```python
from build123d import *

# Parameters (mm, degrees)
BOSS_EXTRUDE1_DEPTH = 1.3
SKETCH2_W           = 6.25
SKETCH2_H           = 1
CUT_EXTRUDE1_DEPTH  = 128.618193671
SKETCH3_W           = 12
SKETCH3_H           = 1
SKETCH3_W_2         = 30
SKETCH3_W_3         = 14
SKETCH3_W_4         = 1
SKETCH3_H_2         = 8
CUT_EXTRUDE2_DEPTH  = 128.618193671
SKETCH4_W           = 1
SKETCH4_H           = 10
CUT_EXTRUDE3_DEPTH  = 128.618193671
SKETCH5_W           = 25
SKETCH5_H           = 1
SKETCH5_W_2         = 1
SKETCH5_H_2         = 20
CUT_EXTRUDE4_DEPTH  = 128.618193671
SKETCH6_W           = 1
SKETCH6_H           = 10
CUT_EXTRUDE5_DEPTH  = 128.618193671
SKETCH7_W           = 24
SKETCH7_H           = 0.5
SKETCH7_W_2         = 86
SKETCH7_W_3         = 18
BOSS_EXTRUDE2_DEPTH = 1.3
CUT_EXTRUDE6_DEPTH  = 128.618193671
SKETCH10_W          = 1
SKETCH10_H          = 40.53071679
BOSS_EXTRUDE3_DEPTH = 1.3


with BuildPart() as part:
    # Sketch1 → Boss-Extrude1 (new body)
    with BuildSketch(Plane(origin=(0, 0, 0), x_dir=(0, 0, -1), z_dir=(1, 0, 0))):
        with BuildLine():
            Line((81.367510562, 0), (81.367510562, 40))
            Line((81.367510562, 40), (68.86751224, 40))
            Line((68.86751224, 40), (68.86751224, 31.6))
            ThreePointArc((68.86751224, 31.6), (60.650673838, 32.5501447), (52.86751224, 35.350431081))
            ThreePointArc((52.86751224, 35.350431081), (27.570153703, 44.311585339), (0.86751224, 47))
            ThreePointArc((0.86751224, 47), (-29.363130095, 42.186071485), (-57.13248776, 29.304750955))
            ThreePointArc((-57.13248776, 29.304750955), (-60.244560512, 27.872141345), (-63.63248776, 27.362910487))
            ThreePointArc((-63.63248776, 27.362910487), (-91.690071427, 24.380332585), (-118.63248776, 16))
            ThreePointArc((-118.63248776, 16), (-117.739294054, 7.999999906), (-118.632489438, 0))
            Line((-118.632489438, 0), (-94.632489438, 0))
            ThreePointArc((-94.632489438, 0), (-76.632489438, 18), (-58.632489438, 0))
            Line((-58.632489438, 0), (27.367510562, 0))
            ThreePointArc((27.367510562, 0), (45.367510562, 18), (63.367510562, 0))
            Line((63.367510562, 0), (81.367510562, 0))
        make_face()
        with BuildLine():
            Line((-42.73248776, 29.304750955), (-2.13248776, 29.304750955))
            Line((-2.13248776, 29.304750955), (-2.13248776, 40.804750955))
            ThreePointArc((-2.13248776, 40.804750955), (-23.231125157, 37.874288199), (-42.73248776, 29.304750955))
        make_face(mode=Mode.SUBTRACT)
    extrude(amount=BOSS_EXTRUDE1_DEPTH)

    # Sketch2 → Cut-Extrude1 (cut, through all)
    with BuildSketch(Plane(origin=(1.3, 0, 0), x_dir=(0, 0, -1), z_dir=(1, 0, 0))):
        with Locations((75.242510562, 38)):
            Rectangle(SKETCH2_W, SKETCH2_H)
    extrude(amount=-CUT_EXTRUDE1_DEPTH, mode=Mode.SUBTRACT)

    # Sketch3 → Cut-Extrude2 (cut, through all)
    with BuildSketch(Plane(origin=(1.3, 0, 0), x_dir=(0, 0, -1), z_dir=(1, 0, 0))):
        with Locations((73.117510562, 1.75)):
            Rectangle(SKETCH3_W, SKETCH3_H)
        with Locations((6.367510562, 1.75)):
            Rectangle(SKETCH3_W_2, SKETCH3_H)
        with Locations((-105.632489438, 1.75)):
            Rectangle(SKETCH3_W_3, SKETCH3_H)
        Polygon((-90.165047606, 22.486285602), (-72.411906778, 25.457142507), (-72.246859172, 24.470856905), (-90, 21.5), align=None)
        with Locations((-107.132489438, 10.75)):
            Rectangle(SKETCH3_W_4, SKETCH3_H_2)
        Polygon((39.458953443, 39.317791271), (59.607847956, 30.484782164), (59.206347542, 29.568923322), (39.057453029, 38.40193243), align=None)
        with Locations((-33.632489438, 1.75)):
            Rectangle(SKETCH3_W_2, SKETCH3_H)
    extrude(amount=-CUT_EXTRUDE2_DEPTH, mode=Mode.SUBTRACT)

    # Sketch4 → Cut-Extrude3 (cut, through all)
    with BuildSketch(Plane(origin=(1.3, 0, 0), x_dir=(0, 0, -1), z_dir=(1, 0, 0))):
        with Locations((79.367510562, 15.75)):
            Rectangle(SKETCH4_W, SKETCH4_H)
    extrude(amount=-CUT_EXTRUDE3_DEPTH, mode=Mode.SUBTRACT)

    # Sketch5 → Cut-Extrude4 (cut, through all)
    with BuildSketch(Plane(origin=(1.3, 0, 0), x_dir=(0, 0, -1), z_dir=(1, 0, 0))):
        with Locations((3.867510562, 43.75)):
            Rectangle(SKETCH5_W, SKETCH5_H)
        with Locations((5.867510562, 22)):
            Rectangle(SKETCH5_W_2, SKETCH5_H_2)
    extrude(amount=-CUT_EXTRUDE4_DEPTH, mode=Mode.SUBTRACT)

    # Sketch6 → Cut-Extrude5 (cut, through all)
    with BuildSketch(Plane(origin=(1.3, 0, 0), x_dir=(0, 0, -1), z_dir=(1, 0, 0))):
        with Locations((-47.132489438, 12.25)):
            Rectangle(SKETCH6_W, SKETCH6_H)
    extrude(amount=-CUT_EXTRUDE5_DEPTH, mode=Mode.SUBTRACT)

    # Sketch7 → Boss-Extrude2 (add)
    with BuildSketch(Plane(origin=(0, 0, 0), x_dir=(0, 0, -1), z_dir=(1, 0, 0))):
        with Locations((-106.632489438, -0.25)):
            Rectangle(SKETCH7_W, SKETCH7_H)
        with Locations((-15.632489438, -0.25)):
            Rectangle(SKETCH7_W_2, SKETCH7_H)
        with Locations((72.367510562, -0.25)):
            Rectangle(SKETCH7_W_3, SKETCH7_H)
    extrude(amount=BOSS_EXTRUDE2_DEPTH)

    # Sketch9 → Cut-Extrude6 (cut, through all)
    with BuildSketch(Plane(origin=(1.3, 0, 0), x_dir=(0, 0, -1), z_dir=(1, 0, 0))):
        with BuildLine():
            Line((15.86751224, 40.804750955), (15.86751224, 29.304750955))
            Line((15.86751224, 29.304750955), (45.86751224, 29.304750955))
            ThreePointArc((45.86751224, 29.304750955), (31.931836066, 37.831247893), (15.86751224, 40.804750955))
        make_face()
    extrude(amount=-CUT_EXTRUDE6_DEPTH, mode=Mode.SUBTRACT)

    # Sketch10 → Boss-Extrude3 (add)
    with BuildSketch(Plane(origin=(0, 0, 0), x_dir=(0, 0, -1), z_dir=(1, 0, 0))):
        with Locations((81.867510562, 19.734641605)):
            Rectangle(SKETCH10_W, SKETCH10_H)
    extrude(amount=BOSS_EXTRUDE3_DEPTH)


solid = part.part
```
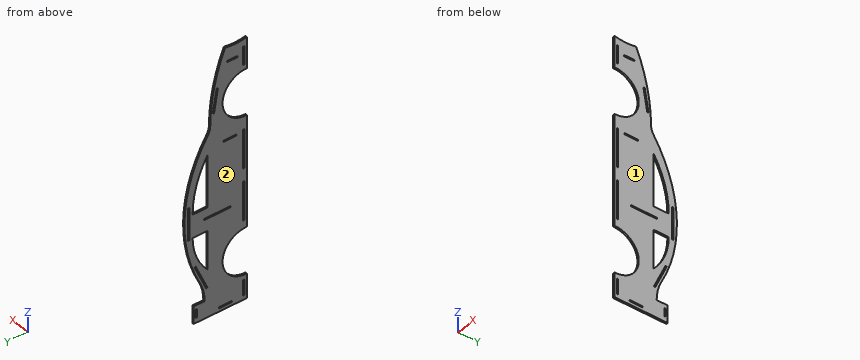
Work out the finished part from the listing and answer in its coordinate system (mm). Face numbers are marked on the shaded views. Round coordinates to 2 decimals unless told otherwise and drop trailing zeros. Write each loop counter-clockwise with the first axis right and the second up, starting at its lowest first coordinate (ties: lowest second). Pieces come first, ordered by that corner, then holes.
1) A cutting plane is placed at B-B on z = -35. Determine the outline of the cut face in (x, y), and give its area (3 significant figures).
2) Determine the mould class of the marked faces 1 and 2 for opening direction X: pulls with the +X half, pulls with the -X half, needs draft (parallel to the pull), parting line crosses it, or undercut.
3) Flat-ended cylindrical pins translate along their axes: P1, Ø0.6, axis at x = 1, z = -76, coming from the -Y side; P2, Ø0.5, axis at x = 0.5, y = 2, coming from the +Z side; P3, Ø0.6, axis at x = 0.5, y = 36.5, coming from the +Z side. Find the tip coordinate at first contact, or state that the pin passes through.
4) Consider probe 1 along Y at (x, z) = (0.55, 30); probe 2 along Z at (x, y) = (0.95, 4.5); probe 3 along Z at (x, y) = (1.1, 5). Determine where each line is inside the solid, lowest interval first.
5) A cutting plane is placed at D-D on z = 81.5. Determine the outline of the cut face in (x, y), and give its area (3 significant figures).
6) A cutting plane is placed at C-C on x = 0.3. Give the number of separate pieces and of enclosed holes in the cut face, and give its area (3 significant figures).
7) A cutting plane is placed at A-A on z = 33.5. Determine the outline of the cut face in (x, y).
Entries:
1. outline: (0, 14.71) - (1.3, 14.71) - (1.3, 29.3) - (0, 29.3) - close; (0, 36.52) - (1.3, 36.52) - (1.3, 42.38) - (0, 42.38) - close
1. area: 26.6 mm2
2. face 1: pulls with the +X half
2. face 2: pulls with the -X half
3. P1: stops at y = -0.5
3. P2: stops at z = 118.28
3. P3: stops at z = 44.77
4. probe 1: y = -0.5 to 1.25, 2.25 to 29.3, 35.62 to 41.99
4. probe 2: z = -82.37 to -62.8, -27.94 to 59.2, 94.06 to 117.91
4. probe 3: z = -82.37 to -62.66, -28.08 to 59.34, 93.92 to 117.86
5. outline: (0, 17.33) - (1.3, 17.33) - (1.3, 22.92) - (0, 22.92) - close; (0, 23.94) - (1.3, 23.94) - (1.3, 26.11) - (0, 26.11) - close
5. area: 10.1 mm2
6. separate pieces: 1
6. enclosed holes: 14
6. area: 5,460 mm2
7. outline: (0, -0.5) - (1.3, -0.5) - (1.3, 1.25) - (0, 1.25) - close; (0, 2.25) - (1.3, 2.25) - (1.3, 29.3) - (0, 29.3) - close; (0, 34.17) - (1.3, 34.17) - (1.3, 40.83) - (0, 40.83) - close
